Check sheet for the modelled part. Datum: model origin and axes. Units: mm. Give positions to 0.01 mm unless a question says otherwise; leave off trailing zeros. Write each loop counter-clockwise with the first axis right and the second up, starting at its lowest first coordinate (ties: lowest second). Pieces come first, ordered by that corner, then holes. Notation, with made-up numbers: M 78,84.5 L 87,84.5 A23 ccw 87,98.5 Z; hole C 76,41.25 d11. An arc over 180 degrees is marked long. Write item = value, one per line. Start each with the question number.
1) Cross-section at C-C, the plane x = 69.5. Record the cut outline in (y, z) (3 decimals), plus the area to 3 significant figures.
2) Cross-section at A-A, the plane x = 27. Record the cut outline in (y, z) (3 decimals).
3) Cross-section at B-B, the plane z = -30.5. Record the cut outline in (x, y) (3 decimals).
4) Go/stop test with flat-tipped pins: pin 1 (0.9 mm diameter, centred on y = 548, z = -32, fed in from +X); pin 2 (2 mm diameter, centred on x = 52.17, z = 27.49, fed in from +Y); pin 3 (1.5 mm diameter, centred on x = 40.5, y = 548, fed in from +Z); pin 4 (1.6 mm diameter, centred on x = 27.5, y = 548.5, fed in from +Z). Record where each tip stops, or that it passes through.
5) Cross-section at D-D, the plane y = 547.7. Give the number of separate pieces and of enclosed holes in the cut face, plus the area to 3 significant figures.
6) Scan lines: line 1 along Z through (x, y) = (27.5, 549.65); line 2 along Z through (x, y) = (59.5, 547.15); line 3 along X through (y, z) = (549.5, 13). Record each from-to range of solid material in increasing order. Write a range as [from, to].
```python
from build123d import *

# Parameters (mm, degrees)
BASE_FLANGE1_DEPTH           = 3.125
F_10_5_10_5_DIAMETER_HOLE1_D = 10.5
F_3_2_3_2_DIAMETER_HOLE1_D   = 3.2
F_23_0_23_DIAMETER_HOLE1_D   = 23
F_6_0_6_DIAMETER_HOLE1_D     = 6
F_2_5_2_5_DIAMETER_HOLE1_D   = 2.5


# Sheet-metal steps are written as plain solids
with BuildPart() as part:
    # Sketch11 → Base-Flange1 (new body)
    with BuildSketch(Plane.XZ.offset(-546.875)):
        with BuildLine():
            Line((22.410254546, -39.506758362), (32.373254546, -39.506758362))
            ThreePointArc((32.373254546, -39.506758362), (35.767367096, -38.100870912), (37.173254546, -34.706758362))
            Line((37.173254546, -34.706758362), (37.173254546, -27.506758362))
            ThreePointArc((37.173254546, -27.506758362), (38.63772064, -23.971224456), (42.173254546, -22.506758362))
            Line((42.173254546, -22.506758362), (75.173254546, -22.506758362))
            ThreePointArc((75.173254546, -22.506758362), (78.708788452, -21.042292268), (80.173254546, -17.506758362))
            Line((80.173254546, -17.506758362), (80.173254546, 20.461534485))
            ThreePointArc((80.173254546, 20.461534485), (80.043518399, 21.59313954), (79.661042546, 22.666020563))
            ThreePointArc((79.661042546, 22.666020563), (78.493233643, 24.758111736), (77.112510881, 26.71623016))
            ThreePointArc((77.112510881, 26.71623016), (75.461078133, 31.260231972), (70.735506318, 32.282070323))
            ThreePointArc((70.735506318, 32.282070323), (52.617226801, 34.461366888), (38.694730703, 22.663676919))
            ThreePointArc((38.694730703, 22.663676919), (38.312910767, 21.593045514), (38.182772618, 20.463841312))
            Line((38.182772618, 20.463841312), (38.16624905, 0.493241638))
            Line((38.16624905, 0.493241638), (22.410254546, 0.493241638))
            ThreePointArc((22.410254546, 0.493241638), (19.016141997, -0.912645812), (17.610254546, -4.306758362))
            Line((17.610254546, -4.306758362), (17.610254546, -34.706758362))
            ThreePointArc((17.610254546, -34.706758362), (19.016141997, -38.100870912), (22.410254546, -39.506758362))
        make_face()
    extrude(amount=-BASE_FLANGE1_DEPTH)

    # Ø10.5 (10.5) Diameter Hole1 (through all)
    with Locations(Plane(origin=(0, 546.875, 0), x_dir=(-1, 0, 0), z_dir=(0, -1, 0))):
        with Locations((-62.173254546, -27.493241638)):
            Hole(F_10_5_10_5_DIAMETER_HOLE1_D / 2)

    # Ø3.2 (3.2) Diameter Hole1 (through all)
    with Locations(Plane(origin=(0, 546.875, 0), x_dir=(-1, 0, 0), z_dir=(0, -1, 0))):
        with Locations((-74.664196355, -13.984183447), (-43.682312737, -13.984183447), (-43.682312737, 16.997700171), (-74.664196355, 16.997700171)):
            Hole(F_3_2_3_2_DIAMETER_HOLE1_D / 2)

    # Ø23.0 (23) Diameter Hole1 (through all)
    with Locations(Plane(origin=(0, 546.875, 0), x_dir=(-1, 0, 0), z_dir=(0, -1, 0))):
        with Locations((-59.173254546, 1.506758362)):
            Hole(F_23_0_23_DIAMETER_HOLE1_D / 2)

    # Ø6.0 (6) Diameter Hole1 (through all)
    with Locations(Plane(origin=(0, 546.875, 0), x_dir=(-1, 0, 0), z_dir=(0, -1, 0))):
        with Locations((-27.173254546, 9.506758362), (-27.173254546, 29.506758362)):
            Hole(F_6_0_6_DIAMETER_HOLE1_D / 2)

    # Ø2.5 (2.5) Diameter Hole1 (through all)
    with Locations(Plane(origin=(0, 546.875, 0), x_dir=(-1, 0, 0), z_dir=(0, -1, 0))):
        with Locations((-72.173254546, -27.493241653), (-52.173254546, -27.493241653)):
            Hole(F_2_5_2_5_DIAMETER_HOLE1_D / 2)


solid = part.part
```
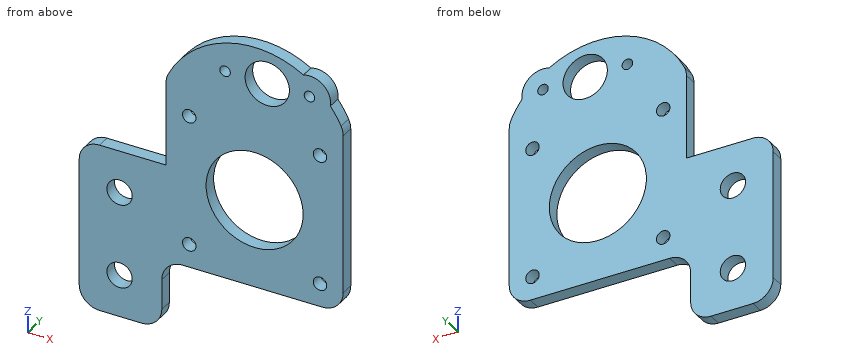
Reply:
q1.outline = M 546.875,-22.507 L 550,-22.507 L 550,-6.567 L 546.875,-6.567 Z; M 546.875,3.554 L 550,3.554 L 550,32.957 L 546.875,32.957 Z
q1.area = 142 mm2
q2.outline = M 546.875,-39.507 L 550,-39.507 L 550,-32.502 L 546.875,-32.502 Z; M 546.875,-26.512 L 550,-26.512 L 550,-12.502 L 546.875,-12.502 Z; M 546.875,-6.512 L 550,-6.512 L 550,0.493 L 546.875,0.493 Z
q3.outline = M 17.61,546.875 L 24.342,546.875 L 24.342,550 L 17.61,550 Z; M 30.004,546.875 L 37.173,546.875 L 37.173,550 L 30.004,550 Z
q4.pin_1 = 37.17
q4.pin_2 = through
q4.pin_3 = 26.72
q4.pin_4 = 0.49
q5.separate_pieces = 1
q5.enclosed_holes = 10
q5.area = 2,470 mm2
q6.line_1 = [-39.51, -32.49], [-26.52, -12.49], [-6.52, 0.49]
q6.line_2 = [-22.51, -13], [9.99, 22.97], [32.01, 35.42]
q6.line_3 = [38.18, 42.42], [44.94, 73.4], [75.93, 80.17]
